Study the drawing (mm; zero at the part's minimum x, y, z) and answer. A direction names the side the tool comes from. Coordinates: 2 decimals unless noted, no trailing zeros. Order: outer loops, then holes, each group sorted by start corner. A loop starts at its lowest first (then second) coordinate and runs counter-clockwise, first axis right, second up. Notation, with made-up numbers: (81.25, 8) -> (99.25, 8) arc R11 ccw to (99.25, 23) -> close; hole circle Ø1 at (44, 73). An arc over 180 degrees is marked (long way). Answer in a Markdown table with one row per item. Add a question column.
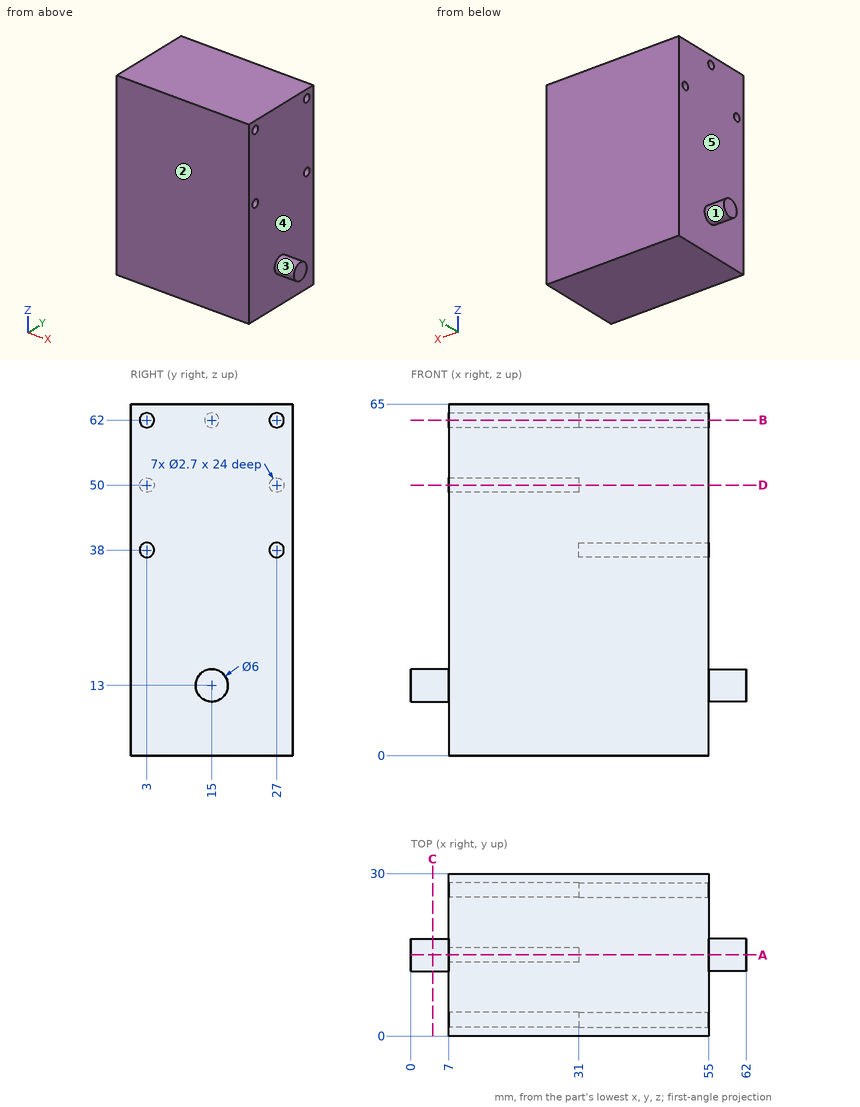
Q1. Straight lines are drawn through the part: line 1 (Y direction, x = 40, z = 38); line 2 (Z direction, x = 23.75, y = 15); line 3 (Y direction, x = 21, z = 62). For each, find the intervals that lie inside material, in ascending order.
Q2. For the marked faces 1 and 2, determine the directions among +Z, -Z, +X, -X, +Y, -Y from which every point of the face is accessible in a straight line to the end or side of a thin tool.
Q3. Given pin 1 (3 mm diameter, centred on y = 15, z = 62, fed in from -X); pin 2 (0.8 mm diameter, centred on y = 26.5, z = 62.5, fed in from +X); pin 3 (15 mm diameter, centred on y = 13.5, z = 40, fed in from +X); pin 4 (12 mm diameter, centred on x = 45, z = 34.5, fed in from -Y), each flat-ended and moving along its own axis, determine where each tip first touches the part or whether it passes through.
Q4. A cutting plane is placed at C-C (x = 4). Determine the outline of the cut face in (y, z).
Q5. Determine the mould class of the marked faces 3, 4 and 5 for opening direction X: +X half, -X half, draft (parallel to the pull), parting line (faces both ways), or undercut.
Q6. A cutting plane is placed at D-D (z = 50). Determine the outline of the cut face in (x, y).
Q7. A cutting plane is placed at A-A (y = 15). Determine the outline of the cut face in (x, z), then the cut area to 3 significant figures.
Q8. A cutting plane is placed at B-B (z = 62). Determine the outline of the cut face in (x, y).
Returned:
| question | item | result |
|---|---|---|
| 1 | line 1 | y = 0 to 1.65, 4.35 to 25.65, 28.35 to 30 |
| 1 | line 2 | z = 0 to 60.65, 63.35 to 65 |
| 1 | line 3 | y = 0 to 13.65, 16.35 to 30 |
| 2 | face 1 | -X |
| 2 | face 2 | +Z, -Z, +X, -X, -Y |
| 3 | pin 1 | stops at x = 7 |
| 3 | pin 2 | stops at x = 31 |
| 3 | pin 3 | stops at x = 55 |
| 3 | pin 4 | stops at y = 0 |
| 4 | outline | circle Ø6 at (15, 13) |
| 5 | face 3 | draft |
| 5 | face 4 | +X half |
| 5 | face 5 | -X half |
| 6 | outline | (7, 0) -> (55, 0) -> (55, 30) -> (7, 30) -> (7, 28.35) -> (31, 28.35) -> (31, 25.65) -> (7, 25.65) -> (7, 4.35) -> (31, 4.35) -> (31, 1.65) -> (7, 1.65) -> close |
| 7 | outline | (0, 10) -> (7, 10) -> (7, 0) -> (55, 0) -> (55, 10) -> (62, 10) -> (62, 16) -> (55, 16) -> (55, 65) -> (7, 65) -> (7, 63.35) -> (31, 63.35) -> (31, 60.65) -> (7, 60.65) -> (7, 16) -> (0, 16) -> close |
| 7 | area | 3,140 mm² |
| 8 | outline | (7, 0) -> (55, 0) -> (55, 1.65) -> (31, 1.65) -> (31, 4.35) -> (55, 4.35) -> (55, 25.65) -> (31, 25.65) -> (31, 28.35) -> (55, 28.35) -> (55, 30) -> (7, 30) -> (7, 16.35) -> (31, 16.35) -> (31, 13.65) -> (7, 13.65) -> close |
